Could you check a few things on this drawing? It's one solid part, dimensions in mm from its lowest x, y, z. A direction names the side the tool comes from. Coordinates: 2 decimals unless noted, no trailing zeros. Order: outer loops, then holes, each group sorted by start corner. A loop starts at its lowest first (then second) coordinate and runs counter-clockwise, first axis right, second up.
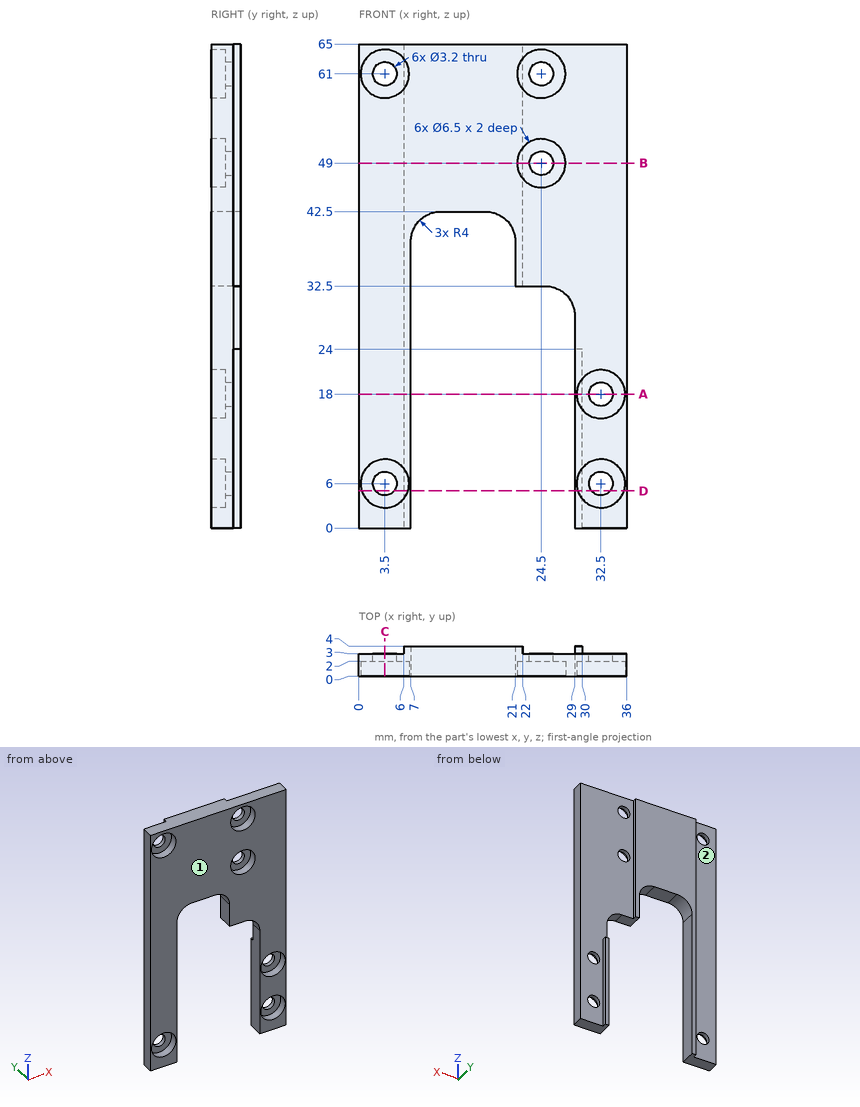
Item 1: Suppose I cut it at D-D (z = 5). List the corners of the cut face in (x, y) for me, and give its area (3 significant figures).
Item 2: Which directions (+Z, -Z, +X, -X, +Y, -Y) give clear straight access to the entire face, cutting with the end or side of a thin tool? Please do the marked faces 1 and 2.
Item 3: Suppose I cut it at B-B (z = 49). List the corners of the cut face in (x, y) for me, and give its area (3 significant figures).
Item 4: For pin 1 Ø4 at (x, z) = (24.5, 61) entering from +Y; pin 2 Ø5 at (x, z) = (24.5, 61) entering from -Y, each with a flat end and sliding along its axis, tell me the tip position at first contact or that it passes through.
Item 5: I need wall thicknesses on line 1 (Z direction, x = 24.5, y = 2.75); line 2 (X direction, y = 0.6, z = 6); line 3 (Z direction, x = 3.5, y = 0.9). Which ranges of each line are inside material? Lowest first, please.
Item 6: Suppose I cut it at C-C (x = 3.5). List the corners of the cut face in (y, z) for me, and give its area (3 significant figures).
Item 7: Suppose I cut it at A-A (z = 18). List the corners of the cut face in (x, y) for me.
Geometry results:
1. outline: (0, 0) - (0.41, 0) - (0.41, 2) - (2.25, 2) - (2.25, 3) - (0, 3) - close; (4.75, 2) - (6.59, 2) - (6.59, 0) - (7, 0) - (7, 4) - (6, 4) - (6, 3) - (4.75, 3) - close; (29, 0) - (29.41, 0) - (29.41, 2) - (31.25, 2) - (31.25, 3) - (30, 3) - (30, 4) - (29, 4) - close; (33.75, 2) - (35.59, 2) - (35.59, 0) - (36, 0) - (36, 3) - (33.75, 3) - close
1. area: 14.3 mm2
2. face 1: +Z, -Z, +X, -X, -Y
2. face 2: +Z, -Z, -X, +Y
3. outline: (0, 0) - (21.25, 0) - (21.25, 2) - (22.9, 2) - (22.9, 3) - (22, 3) - (22, 4) - (6, 4) - (6, 3) - (0, 3) - close; (26.1, 2) - (27.75, 2) - (27.75, 0) - (36, 0) - (36, 3) - (26.1, 3) - close
3. area: 108 mm2
4. pin 1: stops at y = 3
4. pin 2: stops at y = 2
5. line 1: z = 32.5 to 47.4, 50.6 to 59.4, 62.6 to 65
5. line 2: x = 0 to 0.25, 6.75 to 7, 29 to 29.25, 35.75 to 36
5. line 3: z = 0 to 2.75, 9.25 to 57.75, 64.25 to 65
6. outline: (0, 0) - (3, 0) - (3, 4.4) - (2, 4.4) - (2, 2.75) - (0, 2.75) - close; (0, 9.25) - (2, 9.25) - (2, 7.6) - (3, 7.6) - (3, 59.4) - (2, 59.4) - (2, 57.75) - (0, 57.75) - close; (0, 64.25) - (2, 64.25) - (2, 62.6) - (3, 62.6) - (3, 65) - (0, 65) - close
6. area: 163 mm2
7. outline: (0, 0) - (7, 0) - (7, 4) - (6, 4) - (6, 3) - (0, 3) - close; (29, 0) - (29.25, 0) - (29.25, 2) - (30.9, 2) - (30.9, 3) - (30, 3) - (30, 4) - (29, 4) - close; (34.1, 2) - (35.75, 2) - (35.75, 0) - (36, 0) - (36, 3) - (34.1, 3) - close
